```python
from build123d import *

# Parameters (mm, degrees)
F0_R      = 76.2
F1_DEPTH  = 19.05
F2_W      = 25.4
F2_H      = 19.05
F3_DEPTH  = 8.89
F4_R      = 6.604
F5_DEPTH  = 10.16
F6_R      = 3.175
F7_DEPTH  = 19.05
F8_R      = 3.175
F8_R_2    = 19.05
F9_DEPTH  = 19.05
F10_R     = 3.175
F10_R_2   = 19.05
F11_DEPTH = 19.05


with BuildPart() as f1:
    # F0 (on Top) → F1 (new body)
    with BuildSketch(Plane.XY):
        Circle(F0_R)
    extrude(amount=F1_DEPTH)

    # F2 (on face) → F3 (cut)
    with BuildSketch(Plane.XY.offset(19.05)):
        with Locations((-38.1, 0)):
            Rectangle(F2_W, F2_H)
    extrude(amount=-F3_DEPTH, mode=Mode.SUBTRACT)

    # F4 (on face) → F5 (cut)
    with BuildSketch(Plane(origin=(0, 0, 0), x_dir=(1, 0, 0), z_dir=(0, 0, -1))):
        with Locations((-38.1, 0)):
            Circle(F4_R)
    extrude(amount=-F5_DEPTH, mode=Mode.SUBTRACT)

    # F6 (on face) → F7 (cut)
    with BuildSketch(Plane(origin=(0, 0, 0), x_dir=(1, 0, 0), z_dir=(0, 0, -1))):
        with Locations((0, 63.5)):
            Circle(F6_R)
        with Locations((63.5, 0)):
            Circle(F6_R)
        with Locations((0, -63.5)):
            Circle(F6_R)
        with Locations((-63.5, 0)):
            Circle(F6_R)
    extrude(amount=-F7_DEPTH, mode=Mode.SUBTRACT)

    # F8 (on face) → F9 (join)
    with BuildSketch(Plane(origin=(0, 0, 0), x_dir=(1, 0, 0), z_dir=(0, 0, -1))):
        with BuildLine():
            ThreePointArc((-76.2, -9.238e-07), (-25.3999995381, -50.8), (25.4, 0))
            ThreePointArc((25.4, 0), (-25.4000004619, 50.8), (-76.2, -9.238e-07))
        make_face()
        with Locations((-63.5, 0)):
            Circle(F8_R, mode=Mode.SUBTRACT)
        with Locations((-38.1, 0)):
            Circle(F8_R_2, mode=Mode.SUBTRACT)
    extrude(amount=F9_DEPTH)

    # F10 (on face) → F11 (join)
    with BuildSketch(Plane(origin=(0, 0, -19.05), x_dir=(1, 0, 0), z_dir=(0, 0, -1))):
        with BuildLine():
            ThreePointArc((-76.2, -1.0101e-06), (-38.099999495, -38.1), (0, 0))
            ThreePointArc((0, 0), (-38.100000505, 38.1), (-76.2, -1.0101e-06))
        make_face()
        with Locations((-63.5, 0)):
            Circle(F10_R, mode=Mode.SUBTRACT)
        with Locations((-38.1, 0)):
            Circle(F10_R_2, mode=Mode.SUBTRACT)
    extrude(amount=F11_DEPTH)


solid = f1.part
```
Here's how the part is built. I have some questions about the finished solid (model axes, mm). A direction names the side the tool comes from. Round coordinates to 2 decimals unless told otherwise and drop trailing zeros. Order: outer loops, then holes, each group sorted by start corner. A loop starts at its lowest first (then second) coordinate and runs counter-clockwise, first axis right, second up. Notation, with made-up numbers: M 78.25,48 L 103.25,48 A20 cw 103.25,73 Z; hole C 53,12 d5. An arc over 180 degrees is marked long. One line per question, with ' | ' between items.
1) For faces 4 (the face through (-50.8, 0, 15)), 5 (the face through (-19.93, -5.72, -18.78)), 6 (the face through (1.707, -66.177, 9.392)), which set-ups out of +Z, -Z, +X, -X, +Y, -Y let a thin tool reach every point of the face, with its end or its side?
Working result:
face 4: +Z | face 5: -Z | face 6: +Z, -Z
2) If we mould it in two halves opening along X, with no side actions, what happens to faces 1 (the face through (21.526, 19.457, -9.392)), 2 (the face through (-1, 1, 19.05)), 3 (the face through (-38, -9.525, 15))? For each: +X half, -X half, draft (parallel to the pull), parting line (faces both ways), or undercut.
Working result:
face 1: parting line | face 2: draft | face 3: undercut
3) I want a section at C-C, the plane z = -25.5. Write out the boundary of the cut face in (x, y) (3 decimals), then the cut area to 3 significant figures.
Working result:
outline: C -38.1,0 d76.2; hole C -63.5,0 d6.35; hole C -38.1,0 d38.1 | area: 3,390 mm²
4) I need wall thicknesses on line 1 along X through (y, z) = (-0.5, 9); line 2 along Z through (x, y) = (41, -60.5); line 3 along Y through (x, z) = (63.5, 11.25) (3 decimals). Which ranges of each line are inside material? Lowest first, please.
Working result:
line 1: -76.2 to -66.64, -60.36 to -44.69, -31.51 to 60.36, 66.64 to 76.2 | line 2: 0 to 19.05 | line 3: -42.121 to -3.175, 3.175 to 42.121
5) For pin 1 Ø2 at (y, z) = (-19, 4) entering from +X; pin 2 Ø4.5 at (x, z) = (-44, 14) entering from +Y; pin 3 Ø1.5 at (x, z) = (-59, 3) entering from -Y; pin 4 Ø5 at (x, y) = (0, 63.5) entering from +Z, each with a flat end and sliding along its axis, tell me the tip position at first contact or that it passes through.
Working result:
pin 1: x = 74.04 | pin 2: y = 63.74 | pin 3: y = -49.13 | pin 4: through
6) I want a section at B-B, the plane x = 64. Write out the boundary of the cut face in (y, z), then the cut area to 3 significant figures.
Working result:
outline: M -41.36,0 L -3.14,0 L -3.14,19.05 L -41.36,19.05 Z; M 3.14,0 L 41.36,0 L 41.36,19.05 L 3.14,19.05 Z | area: 1,460 mm²
7) I want a section at A-A, the plane y = 63.5. Write out the boundary of the cut face in (x, z) (3 decimals), then the cut area to 3 significant figures.
Working result:
outline: M -42.121,0 L -3.175,0 L -3.175,19.05 L -42.121,19.05 Z; M 3.175,0 L 42.121,0 L 42.121,19.05 L 3.175,19.05 Z | area: 1,480 mm²
8) I want a section at D-D, the plane z = 2. Write out the boundary of the cut face in (x, y) (3 decimals).
Working result:
outline: C 0,0 d152.4; hole C -63.5,0 d6.35; hole C -38.1,0 d13.208; hole C 0,-63.5 d6.35; hole C 0,63.5 d6.35; hole C 63.5,0 d6.35
